Can you work these out from the model? Positions are in its coordinate system, mm. Face numbers are marked on the shaded views. Coordinates: 2 decimals unless noted, no trailing zeros. Loops run counter-clockwise (first coordinate to the right, second up) from the corner with the lowest first, then second, coordinate; pieces in that order, holes last.
```python
from build123d import *

# Parameters (mm, degrees)
SKETCH1_R           = 4.025
BOSS_EXTRUDE1_DEPTH = 7.5


with BuildPart() as part:
    # Sketch1 → Boss-Extrude1 (new body)
    with BuildSketch(Plane.XY):
        with BuildLine():
            Line((0, -6), (45.64, -6))
            ThreePointArc((45.64, -6), (51.64, 0), (45.64, 6))
            ThreePointArc((45.64, 6), (36.145582493, 8.39727191), (28.927235025, 15.01439638))
            ThreePointArc((28.927235025, 15.01439638), (22.82, 18.308467551), (16.712764975, 15.01439638))
            ThreePointArc((16.712764975, 15.01439638), (9.494417507, 8.39727191), (0, 6))
            ThreePointArc((0, 6), (-6, 0), (0, -6))
        make_face()
        Circle(SKETCH1_R, mode=Mode.SUBTRACT)
        with Locations((45.64, 0)):
            Circle(SKETCH1_R, mode=Mode.SUBTRACT)
        with Locations((22.82, 11)):
            Circle(SKETCH1_R, mode=Mode.SUBTRACT)
    extrude(amount=BOSS_EXTRUDE1_DEPTH)


solid = part.part
```
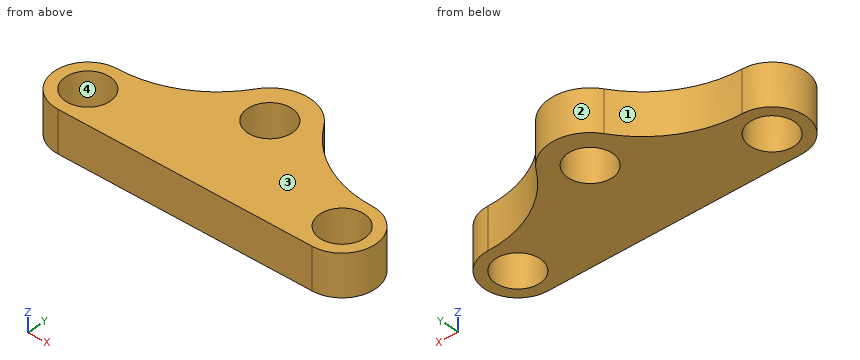
(1) I want a section at D-D on y = 9. Write out the boundary of the cut face in (x, z), then the cut area to 3 significant figures.
Check values:
outline: (10.54, 0) - (19.33, 0) - (19.33, 7.5) - (10.54, 7.5) - close; (26.31, 0) - (35.1, 0) - (35.1, 7.5) - (26.31, 7.5) - close
area: 132 mm2
(2) I want a section at C-C on z = 1.25. Write out the boundary of the cut face in (x, y) (3 decimals), then the cut area to 3 significant figures.
Check values:
outline: (0, -6) - (45.64, -6) arc R6 ccw to (45.64, 6) arc R20 cw to (28.927, 15.014) arc R7.308 ccw to (16.713, 15.014) arc R20 cw to (0, 6) arc R6 ccw to start; hole circle Ø8.05 at (0, 0); hole circle Ø8.05 at (22.82, 11); hole circle Ø8.05 at (45.64, 0)
area: 736 mm2
(3) If I drill on probe 1 along Y at (x, z) = (22.82, 2) (3 decimals); probe 2 along X at (y, z) = (1.25, 4); probe 3 along Y at (x, z) = (45.64, 4.5) (3 decimals), over which ranges is the centre line in solid material (lowest first)?
Check values:
probe 1: y = -6 to 6.975, 15.025 to 18.308
probe 2: x = -5.87 to -3.83, 3.83 to 41.81, 49.47 to 51.51
probe 3: y = -6 to -4.025, 4.025 to 6
(4) I'm going to push flat-ended pins straight in: pin 1 (1 mm diameter, centred on y = 15, z = 1.5, fed in from +X); pin 2 (1 mm diameter, centred on y = 3.5, z = 2, fed in from -X); pin 3 (6.5 mm diameter, centred on x = 22.82, y = 11, fed in from +Z); pin 4 (1.5 mm diameter, centred on y = 12.5, z = 3, fed in from +X). Where does each tip first touch, or does it pass through?
Check values:
pin 1: stops at x = 29.28
pin 2: stops at x = -5.2
pin 3: passes through
pin 4: stops at x = 31.61
(5) If we mould it in two halves opening along X, with no side actions, what happens to the marked faces 1, 2, 3 and 4? For each: released by +X, released by -X, zero draft, split by the parting line, or undercut.
Check values:
face 1: released by -X
face 2: split by the parting line
face 3: zero draft
face 4: undercut
(6) I want a section at A-A on y = 0. Write out the boundary of the cut face in (x, z) (3 decimals).
Check values:
outline: (-6, 0) - (-4.025, 0) - (-4.025, 7.5) - (-6, 7.5) - close; (4.025, 0) - (41.615, 0) - (41.615, 7.5) - (4.025, 7.5) - close; (49.665, 0) - (51.64, 0) - (51.64, 7.5) - (49.665, 7.5) - close
(7) I want a section at B-B on x = 22.82. Write out the boundary of the cut face in (y, z) (3 decimals).
Check values:
outline: (-6, 0) - (6.975, 0) - (6.975, 7.5) - (-6, 7.5) - close; (15.025, 0) - (18.308, 0) - (18.308, 7.5) - (15.025, 7.5) - close
